Source: CAD feature listing. Evaluate the final solid. Frame: model axes, mm. A direction names the side the tool comes from. Round coordinates to 2 decimals unless told otherwise and drop trailing zeros. Loops run counter-clockwise (first coordinate to the right, second up) from the corner with the lowest first, then second, coordinate; pieces in that order, holes last. Notation, with made-up numbers: M 15,34 L 54,34 A19 ccw 54,48 Z; hole C 84,57.5 d1. An arc over 180 degrees is marked long. One line per item, written item: value.
Autodesk Inventor part; units mm, degrees
ref_plane "Work Plane1" through (-13.7, -13.7, -46.5) normal (0, 0, -1) x (0, 1, 0)
ref_plane "Work Plane2" through (-18.1, -4, -51.2) normal (0, 0, -1) x (0, 1, 0)
ref_plane "YZ Plane" through (0, 0, 0) normal (1, 0, 0) x (0, 1, 0)
sketch "Sketch1" plane through (0, 0, 0) normal (0, 0, 1) x (1, 0, 0)
  circle A0 centre (0, 0) radius 13.7
  line L0 (18.375, 15.375) -> (-18.1, 15.375)
  line L1 (-18.1, 15.375) -> (-18.1, -4)
  line L2 (-18.1, -4) -> (-13.1031, -4)
  arc A1 (13.1031, -4) -> (-13.1031, -4) centre (0, 0) ccw
  line L3 (13.1031, -4) -> (18.375, -4)
  line L4 (18.375, -4) -> (18.375, 15.375)
  line L5 (18.375, -4) -> (-18.1, -4)
  line L6 (-18.1, -4) -> (-18.1, -15.125)
  line L7 (-18.1, -15.125) -> (18.375, -15.125)
  line L8 (18.375, -15.125) -> (18.375, -4)
  circle A2 centre (44.375, 8.875) radius 25
  point P0 (0, -13.7)
  point P1 (44.375, -16.125)
  dimension "d2" = 29.075
  dimension "d15" = 1
ref_plane "Work Plane1" through (-13.7, -13.7, -46.5) normal (0, 0, -1) x (0, 1, 0)
extrude "Extrusion1" add sketch "Sketch1" against normal up to surface (46.5 mm away) contours A0 L3 L8 L7 L6 L2
sketch "Sketch2" plane through (18.375, -15.125, -46.5) normal (0, 0, -1) x (-1, 0, 0)
  circle A0 centre (26.375, 15.2) radius 1.0564
  circle A1 centre (10.375, 15.2) radius 1.0564
  circle A2 centre (18.375, 15.2) radius 5
  circle A3 centre (18.375, 15.2) radius 13.7
  arc A4 (23.2981, 11.2) -> (13.4519, 11.2) centre (18.375, 15.2) ccw
  circle A5 centre (18.375, 15.2) radius 6.3433
  line L0 (36.475, 0) -> (0, 0)
  line L1 (0, 11.125) -> (5.2719, 11.125)
  line L2 (36.475, 0) -> (0, 0)
  line L3 (0, 0) -> (0, 11.125)
  line L4 (0, 11.125) -> (36.475, 11.125)
  line L5 (36.475, 11.125) -> (36.475, 0)
  point P0 (18.375, 15.125)
  point P1 (23.2362, 11.125)
  point P2 (13.5138, 11.125)
ref_plane "Work Plane2" through (-18.1, -4, -51.2) normal (0, 0, -1) x (0, 1, 0)
extrude "Extrusion2" add sketch "Sketch2" along normal up to surface (4.7 mm away) contours A5 L4 A3 | A3 L4 L5 L0 L3 L1
sketch "Sketch3" plane through (-18.1, -15.125, 0) normal (0, -1, 0) x (1, 0, 0)
  circle A0 centre (33.975, -2.5) radius 1.8
  circle A1 centre (33.975, -48.7) radius 1.8
  circle A2 centre (2.5, -48.7) radius 1.8
  circle A3 centre (2.5, -2.5) radius 1.8
  point P0 (18.1, 0)
hole "Hole1" at (15.875, -15.125, -2.5) at (15.875, -15.125, -48.7) at (-15.6, -15.125, -48.7) at (-15.6, -15.125, -2.5) direction (0, 1, 0) diameter 3.6 end through all countersink diameter 6.5 countersink angle 90
properties part number "right_motor_mount_ceil"
1. Reachability of faces 4 (the face through (-0.078, -6.268, -48.817)), 5 (the face through (0, -9, -46.5)) from +Z, -Z, +X, -X, +Y, -Y: full face, straight path, thin tool, end or side. Return the list, or none.
Report:
face 4: +Z, -Z, +Y
face 5: +Z, +Y
2. Section query A-A (z = -2.5). Return the cut outline in (x, y) (3 decimals).
Report:
outline: M -18.1,-14.375 L -17.4,-13.675 L -17.4,-4 L -18.1,-4 Z; M -13.8,-13.675 L -12.35,-15.125 L 12.625,-15.125 L 14.075,-13.675 L 14.075,-4 L 13.103,-4 A13.7 cw -13.103,-4 L -13.8,-4 Z; M 17.675,-13.675 L 18.375,-14.375 L 18.375,-4 L 17.675,-4 Z
3. Section query B-B (y = -5). Return the cut outline in (x, z) (1 decimal).
Report:
outline: M -18.1,-51.2 L -3.8,-51.2 L -3.8,-46.5 L -12.8,-46.5 L -12.8,0 L -18.1,0 Z; M 3.8,-51.2 L 18.4,-51.2 L 18.4,0 L 12.8,0 L 12.8,-46.5 L 3.8,-46.5 Z; hole C -15.6,-48.7 d3.6; hole C -15.6,-2.5 d3.6; hole C 15.9,-48.7 d3.6; hole C 15.9,-2.5 d3.6
4. Pull-direction query (X, two-part tool) for faces 1 (the face through (-14.21, -13.93, -47.19)), 2 (the face through (18.375, -10, -25)), 3 (the face through (-14, -4, -27)); classes: released by +X, released by -X, zero draft, split by the parting line, or undercut.
Report:
face 1: undercut
face 2: released by +X
face 3: zero draft
5. Ray query, line 1 (Z direction, x = -15.6, y = -10); line 2 (X direction, y = -8.25, z = -48.7) (3 decimals); line 3 (Z direction, x = 17.5, y = -8.75). Return the intervals inside material, ascending. Write a range as [from, to].
Report:
line 1: z = [-51.2, -50.5], [-46.9, -4.3], [-0.7, 0]
line 2: x = [-18.1, -17.4], [-13.8, 14.075], [17.675, 18.375]
line 3: z = [-51.2, -49.47], [-47.93, -3.27], [-1.73, 0]
6. Pin query (flat end, axial travel): pin 1 (6 mm diameter, centred on x = 15.875, z = -48.7, fed in from -Y) (3 decimals); pin 2 (4.5 mm diameter, centred on x = 15.875, z = -2.5, fed in from -Y) (3 decimals); pin 3 (3 mm diameter, centred on x = -1, y = -6.5, fed in from +Z). Return the tip coordinate at first contact, or that it passes through.
Report:
pin 1: stops at y = -14.875
pin 2: stops at y = -14.125
pin 3: stops at z = -46.5
7. Section query C-C (x = -15.6). Return the cut outline in (y, z) (3 decimals).
Report:
outline: M -15.125,-45.45 L -13.675,-46.9 L -4,-46.9 L -4,-4.3 L -13.675,-4.3 L -15.125,-5.75 Z; M -14.375,-51.2 L -4,-51.2 L -4,-50.5 L -13.675,-50.5 Z; M -14.375,0 L -13.675,-0.7 L -4,-0.7 L -4,0 Z
8. Section query D-D (y = -7.25). Return the cut outline in (x, z) (3 decimals).
Report:
outline: M -18.1,-51.2 L 18.375,-51.2 L 18.375,0 L 11.624,0 L 11.624,-46.5 L -11.624,-46.5 L -11.624,0 L -18.1,0 Z; hole C -15.6,-48.7 d3.6; hole C -15.6,-2.5 d3.6; hole C 15.875,-48.7 d3.6; hole C 15.875,-2.5 d3.6
